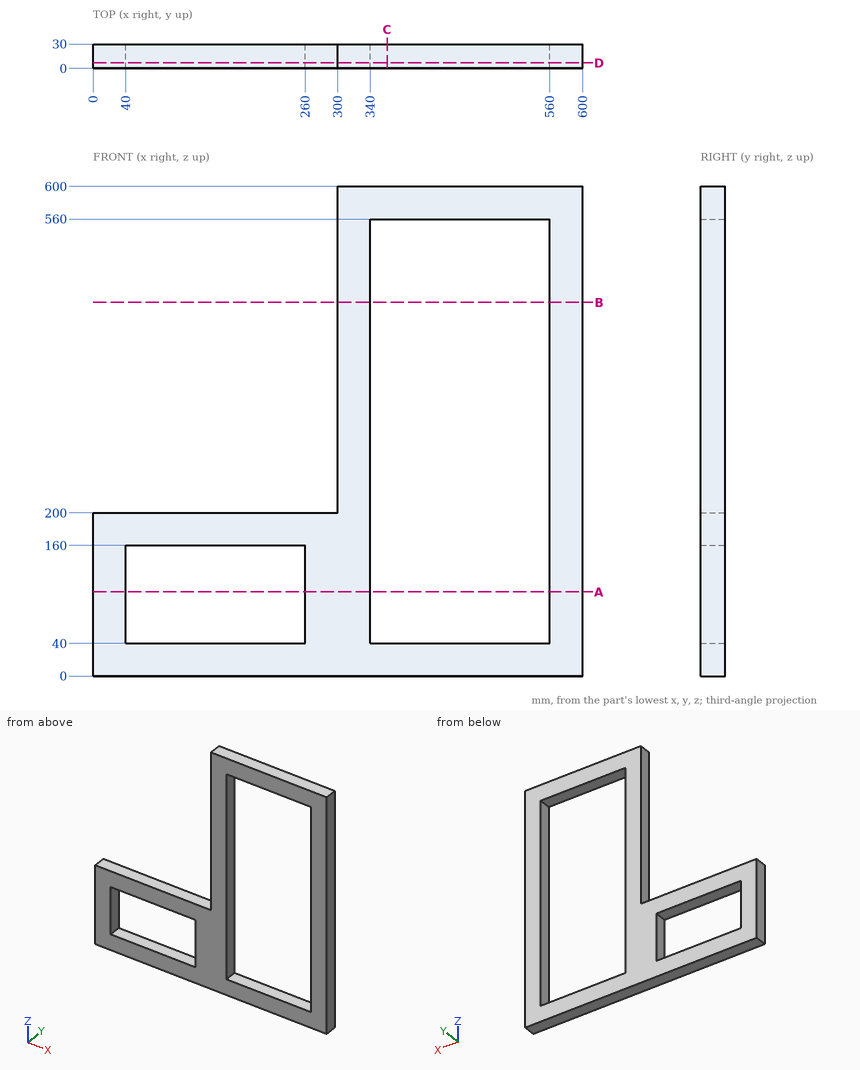
Source: three-view drawing plus pictorial views. Frame: mm from the lowest corner of the part. Give positions to 0.01 mm unless a question says otherwise; leave off trailing zeros. Order: outer loops, then holes, each group sorted by start corner. A loop starts at its lowest first (then second) coordinate and runs counter-clockwise, first axis right, second up. Notation, with made-up numbers: (63.5, 11.5) -> (89.5, 11.5) arc R32 cw to (89.5, 41.5) -> close; hole circle Ø10 at (86.25, -30). An arc over 180 degrees is marked (long way). Use a Markdown table: item, result.
Q1. Section C-C (x = 360.5). Return the cut outline in (y, z), and give its area (3 significant figures).
A:
| item | result |
|---|---|
| outline | (0, 0) -> (30, 0) -> (30, 40) -> (0, 40) -> close; (0, 560) -> (30, 560) -> (30, 600) -> (0, 600) -> close |
| area | 2,400 mm^2 |
Q2. Section A-A (z = 103). Return the cut outline in (x, y).
A:
| item | result |
|---|---|
| outline | (0, 0) -> (40, 0) -> (40, 30) -> (0, 30) -> close; (260, 0) -> (340, 0) -> (340, 30) -> (260, 30) -> close; (560, 0) -> (600, 0) -> (600, 30) -> (560, 30) -> close |
Q3. Section B-B (z = 458). Return the cut outline in (x, y), and give its area (3 significant figures).
A:
| item | result |
|---|---|
| outline | (300, 0) -> (340, 0) -> (340, 30) -> (300, 30) -> close; (560, 0) -> (600, 0) -> (600, 30) -> (560, 30) -> close |
| area | 2,400 mm^2 |
Q4. First-contact query: P1, Ø12, axis at x = 185.5, y = 14, coming from the +Z side; P2, Ø10, axis at y = 15.5, z = 430, coming from the -X side. Flat tips, straight axial feed; report the tip coordinate or a pass-through.
A:
| item | result |
|---|---|
| P1 | z = 200 |
| P2 | x = 300 |
Q5. Section D-D (y = 6.75). Return the cut outline in (x, z).
A:
| item | result |
|---|---|
| outline | (0, 0) -> (600, 0) -> (600, 600) -> (300, 600) -> (300, 200) -> (0, 200) -> close; hole (40, 40) -> (260, 40) -> (260, 160) -> (40, 160) -> close; hole (340, 40) -> (560, 40) -> (560, 560) -> (340, 560) -> close |
Q6. Material intervals for line 1 (X direction, y = 10, z = 127.5); line 2 (X direction, y = 18, z = 237.5); line 3 (Z direction, x = 137.5, y = 14), sorted ascending. Write a range as [from, to].
A:
| item | result |
|---|---|
| line 1 | [0, 40], [260, 340], [560, 600] |
| line 2 | [300, 340], [560, 600] |
| line 3 | [0, 40], [160, 200] |
